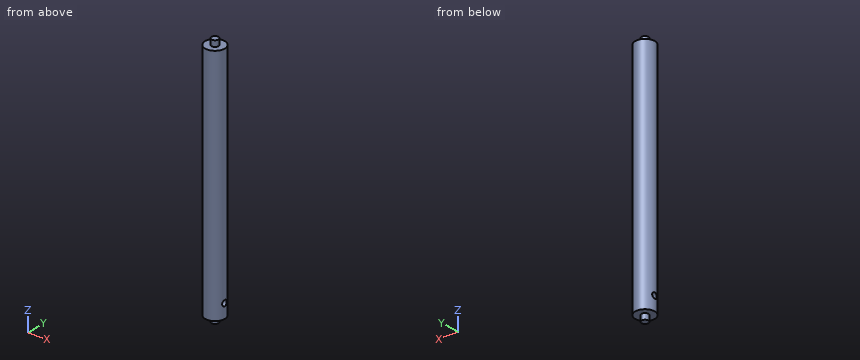
```python
from build123d import *

# Parameters (mm, degrees)
ESQUISSE1_R                  = 50
BOSS_EXTRU_1_DEPTH           = 1215
ESQUISSE2_R                  = 18
BOSS_EXTRU_2_DEPTH           = 30
BOSS_EXTRU_3_START           = 30
ESQUISSE3_R                  = 18
BOSS_EXTRU_3_DEPTH           = 30
ENL_V_MAT_EXTRU_1_DEPTH      = 1248.00641538
ENL_V_MAT_EXTRU_1_DEPTH_BACK = 1248.00641538
ESQUISSE6_R                  = 14.3


with BuildPart() as part:
    # Esquisse1 → Boss.-Extru.1 (new body)
    with BuildSketch(Plane.XY):
        Circle(ESQUISSE1_R)
    extrude(amount=BOSS_EXTRU_1_DEPTH)

    # Esquisse2 → Boss.-Extru.2 (add)
    with BuildSketch(Plane(origin=(0, 0, 0), x_dir=(-1, 0, 0), z_dir=(0, 0, -1))):
        Circle(ESQUISSE2_R)
    extrude(amount=BOSS_EXTRU_2_DEPTH)

    # Esquisse3 → Boss.-Extru.3 (add)
    with BuildSketch(Plane.XY.offset(1215).offset(BOSS_EXTRU_3_START)):
        with Locations(Location((0, 0, 0), (0, 0, 180))):
            Circle(ESQUISSE3_R)
    extrude(amount=-BOSS_EXTRU_3_DEPTH)

    # Esquisse6 → Enlèv. mat.-Extru.1 (cut, two sides: drawn at the far end of the back side and taken through both)
    with BuildSketch(Plane(origin=(0, 0, 0), x_dir=(0, 0, -1), z_dir=(1, 0, 0)).offset(-ENL_V_MAT_EXTRU_1_DEPTH_BACK)):
        with Locations((-71.4, 0)):
            Circle(ESQUISSE6_R)
    extrude(amount=ENL_V_MAT_EXTRU_1_DEPTH + ENL_V_MAT_EXTRU_1_DEPTH_BACK, mode=Mode.SUBTRACT)


solid = part.part
```
Could you check a few things on this model? Use its own coordinates, in mm. Round coordinates to 2 decimals unless told otherwise and drop trailing zeros. Loops run counter-clockwise (first coordinate to the right, second up) from the corner with the lowest first, then second, coordinate; pieces in that order, holes last. Notation, with made-up numbers: (73, 4.25) -> (90, 4.25) arc R17 cw to (90, 34.25) -> close; hole circle Ø9 at (49, 44.5). An arc over 180 degrees is marked (long way). One line per question, with ' | ' between items.
(1) For pin 1 Ø3 at (y, z) = (-28, 588.5) entering from -X; pin 2 Ø3 at (x, z) = (37, 377.5) entering from +Y; pin 3 Ø1 at (x, z) = (-6.5, 926) entering from +Y, each with a flat end and sliding along its axis, tell me the tip position at first contact or that it passes through.
Model answer:
pin 1: stops at x = -42.4 | pin 2: stops at y = 35.21 | pin 3: stops at y = 49.64
(2) If we section it at A-A on y = 0: List the corners of the cut face in (x, z) for me.
Model answer:
outline: (-50, 0) -> (-18, 0) -> (-18, -30) -> (18, -30) -> (18, 0) -> (50, 0) -> (50, 57.1) -> (-50, 57.1) -> close; (-50, 85.7) -> (50, 85.7) -> (50, 1215) -> (18, 1215) -> (18, 1245) -> (-18, 1245) -> (-18, 1215) -> (-50, 1215) -> close
(3) If we section it at C-C on z = 148: List the corners of the cut face in (x, y) for me, and give its area (3 significant figures).
Model answer:
outline: circle Ø100 at (0, 0) | area: 7,850 mm^2
(4) If we section it at B-B on x = 0: List the corners of the cut face in (y, z) for me.
Model answer:
outline: (-50, 0) -> (-18, 0) -> (-18, -30) -> (18, -30) -> (18, 0) -> (50, 0) -> (50, 1215) -> (18, 1215) -> (18, 1245) -> (-18, 1245) -> (-18, 1215) -> (-50, 1215) -> close; hole circle Ø28.6 at (0, 71.4)
(5) If I drill on probe 1 along Z at (x, y) = (24, 0); probe 2 along Z at (x, y) = (-13, 0); probe 3 along X at (y, z) = (-4, 168.5), over which ranges is the centre line in solid material (lowest first)?
Model answer:
probe 1: z = 0 to 57.1, 85.7 to 1215 | probe 2: z = -30 to 57.1, 85.7 to 1245 | probe 3: x = -49.84 to 49.84
